Autodesk Inventor part; units mm, degrees
ref_plane "YZ Plane" through (0, 0, 0) normal (1, 0, 0) x (0, 1, 0)
ref_plane "XZ Plane" through (0, 0, 0) normal (0, 1, 0) x (-1, 0, 0)
ref_plane "XY Plane" through (0, 0, 0) normal (0, 0, 1) x (1, 0, 0)
sketch "Sketch1" plane through (0, 0, 0) normal (0, 1, 0) x (-1, 0, 0)
  circle A0 centre (0, 0) radius 9.75
  circle A1 centre (0, 0) radius 1.5
  circle A2 centre (0, 0) radius 7 construction
  line L0 (0, 0) -> (7, 0) construction
  point P0 (0, 7)
  point P1 (-7, 0)
  point P2 (0, -7)
  dimension "d3" = 14
  dimension "d0" = 19.5
  dimension "d1" = 3
  dimension "d16" = 360
extrude "Extrusion1" add sketch "Sketch1" along normal blind 2.5
sketch "Sketch2" plane through (0, 0, 0) normal (0, -1, 0) x (1, 0, 0)
  circle A0 centre (0, 0) radius 4.375
  circle A1 centre (0, 0) radius 3
  dimension "d10" = 8.75
  dimension "d11" = 6
extrude "Extrusion2" add sketch "Sketch2" along normal blind 2.5
sketch "Sketch3" plane through (0, 0, 0) normal (0, -1, 0) x (1, 0, 0)
  circle A0 centre (0, 0) radius 3
  circle A1 centre (0, 0) radius 1.5
extrude "Extrusion3" cut sketch "Sketch3" against normal blind 1.5
sketch "Sketch4" plane through (0, 2.5, 0) normal (0, 1, 0) x (1, 0, 0)
  circle A0 centre (0, 0) radius 7 construction
  line L0 (0, 7) -> (0, 0) construction
  point P0 (-7, 0)
  point P1 (0, -7)
  point P2 (7, 0)
  dimension "d20" = 14
  dimension "d23" = 360
hole "Hole1" at (-7, 2.5, 0) at (0, 2.5, 7) at (7, 2.5, 0) at (0, 2.5, -7) direction (0, -1, 0) diameter 2.459 end up to surface
properties part number "CH"
Model file for the job. Use its own axes, mm. A direction names the side the tool comes from. Give positions to 0.01 mm unless a question says otherwise; leave off trailing zeros. Loops run counter-clockwise (first coordinate to the right, second up) from the corner with the lowest first, then second, coordinate; pieces in that order, holes last.
Item 1: Slice it at C-C (z = 7). Write the cut outline in (x, y).
Check values:
outline: (-6.79, 0) - (-1.23, 0) - (-1.23, 2.5) - (-6.79, 2.5) - close; (1.23, 0) - (6.79, 0) - (6.79, 2.5) - (1.23, 2.5) - close
Item 2: Drop flat-ended pins along their axis: P1, Ø3.5, axis at x = 0, z = 0, coming from the -Y side; P2, Ø3, axis at y = 1.5, z = 4.5, coming from the -X side. Give the stop position or say it passes through.
Check values:
P1: stops at y = 1.5
P2: stops at x = -9.28
Item 3: Mould opens along X. For faces 1 (the face through (-3, 0, 0)), 2 (the face through (1.269, 1.232, -9.667)), 3 (the face through (-1, -2.5, -3)) say: +X half, -X half, draft (parallel to the pull), parting line (faces both ways), or undercut.
Check values:
face 1: undercut
face 2: parting line
face 3: draft
Item 4: Slice it at B-B (x = -8). Write the cut outline in (y, z), plus the area to 3 significant figures.
Check values:
outline: (0, -5.57) - (2.5, -5.57) - (2.5, -0.72) - (0, -0.72) - close; (0, 0.72) - (2.5, 0.72) - (2.5, 5.57) - (0, 5.57) - close
area: 24.3 mm2
Item 5: Drill centre lines: line 1 along Z through (x, y) = (0, 1.3); line 2 along Z through (x, y) = (0, -1.75) (3 decimals); line 3 along Y through (x, z) = (-7.75, -2.25). Where is each one in solid material? Low to high.
Check values:
line 1: z = -9.75 to -8.23, -5.77 to -3, 3 to 5.77, 8.23 to 9.75
line 2: z = -4.375 to -3, 3 to 4.375
line 3: y = 0 to 2.5
Item 6: Slice it at A-A (z = 0). Give the number of separate pieces and of enclosed holes in the cut face, plus the area to 3 significant figures.
Check values:
separate pieces: 4
enclosed holes: 0
area: 31.3 mm2
Item 7: Slice it at D-D (y = -0.45). Write the cut outline in (x, z) (3 decimals).
Check values:
outline: circle Ø8.75 at (0, 0); hole circle Ø6 at (0, 0)
Item 8: Which spindle directions (+Z, -Z, +X, -X, +Y, -Y) get a long thin tool onto all of the face, cutting with end or side? Do faces 4 (the face through (-2, 2.5, 0)), 5 (the face through (-3.472, -1.232, 2.662)). Say none if no direction does.
Check values:
face 4: +Z, -Z, +X, -X, +Y
face 5: -Y
